```python
from build123d import *

# Parameters (mm, degrees)
F0_W     = 30
F0_H     = 72
F0_R     = 5
F1_DEPTH = 6
F2_R     = 1.25
F3_DEPTH = 1.5
F4_SIZE  = 0.5
F5_SIZE  = 1
F6_R     = 2
F7_W     = 34.31184
F7_H     = 14
F8_DEPTH = 4


with BuildPart() as f1:
    # F0 (on Front) → F1 (new body)
    with BuildSketch(Plane.XZ):
        with Locations((0, -28)):
            Rectangle(F0_W, F0_H)
        with Locations((0, -56)):
            Circle(F0_R, mode=Mode.SUBTRACT)
        with Locations((0, -28)):
            Circle(F0_R, mode=Mode.SUBTRACT)
        Circle(F0_R, mode=Mode.SUBTRACT)
    extrude(amount=-F1_DEPTH)

    # F2 (on Front) → F3 (join)
    with BuildSketch(Plane.XZ):
        with Locations((-13.51, 6.25)):
            Circle(F2_R)
        with Locations((0, -42)):
            Circle(F2_R)
    extrude(amount=F3_DEPTH)

    # F4
    f4_edges = [f1.edges().sort_by_distance(p)[0] for p in [
        (-14.76, -1.5, 6.25),
        (-1.25, -1.5, -42),
    ]]
    chamfer(f4_edges, length=F4_SIZE)

    # F5
    f5_edges = [f1.edges().sort_by_distance(p)[0] for p in [
        (-5, 6, -56),
        (-5, 6, -28),
        (-5, 6, 0),
        (-15, 6, -28),
        (0, 6, -64),
        (0, 6, 8),
        (15, 6, -28),
    ]]
    chamfer(f5_edges, length=F5_SIZE)

    # F6
    f6_edges = [f1.edges().sort_by_distance(p)[0] for p in [
        (-15, 2.5, 8),
        (15, 2.5, 8),
        (15, 2.5, -64),
        (-15, 2.5, -64),
    ]]
    fillet(f6_edges, radius=F6_R)

    # F7 (on Front) → F8 (cut)
    with BuildSketch(Plane.XZ):
        with Locations((5.65592, -14)):
            Rectangle(F7_W, F7_H)
    extrude(amount=-F8_DEPTH, mode=Mode.SUBTRACT)


solid = f1.part
```
Verification items for the finished model (mm, model axes). A direction names the side the tool comes from. Coordinates: 2 decimals unless noted, no trailing zeros. Order: outer loops, then holes, each group sorted by start corner. A loop starts at its lowest first (then second) coordinate and runs counter-clockwise, first axis right, second up. Notation, with made-up numbers: (-15.5, -30.75) -> (1.5, -30.75) arc R17 cw to (1.5, -21.75) -> close; hole circle Ø9 at (-24, -32). An arc over 180 degrees is marked (long way). Put each result on its own line as item: value. Start each with the question number.
1) Cross-section at A-A (z = 0). Enter the section's corners in (x, y).
2) Go/stop test with flat-tipped pins: pin 1 (13 mm diameter, centred on x = 0, z = -56, fed in from +Y); pin 2 (7 mm diameter, centred on x = 4.5, z = -17, fed in from -Y); pin 3 (16 mm diameter, centred on x = 0, z = 0, fed in from -Y). Record where each tip stops, or that it passes through.
3) Release check for a two-part mould opening along X. For faces 3 (the flat face through (0, 2, 8)), 4 (the flat face through (-11.5, 2, -14)), 5 (the cylindrical face through (-0.651, 2.465, -51.043)), 6 (the cylindrical face through (-14.43, 2.83, -63.4)) record: pulls with the +X half, pulls with the -X half, needs draft (parallel to the pull), parting line crosses it, or undercut.
4) Cross-section at C-C (y = 2.25). Enter the section's corners in (x, z).
5) Material ranges on L1, parallel to Z at x = 0, y = 3.25; L2, parallel to Z at x = -2.5, y = 3.5; L3, parallel to Z at x = 10, y = 2.25, recorded low to high.
6) Cross-section at D-D (z = -42). Enter the section's corners in (x, y), plus the area to 4 significant figures.
7) Cross-section at B-B (x = 0). State how many separate pieces and enclosed holes the cut face has, plus the area to 4 significant figures.
8) Tool access check on faces 1 (the flat face through (2, 2, -21)), 2 (the flat face through (0, -1.5, -42)). Record the directions out of +Z, -Z, +X, -X, +Y, -Y that give a thin tool (end or side, any length) a straight path to the whole face; none if there is none.
Geometry check:
1. outline: (-15, 0) -> (-5, 0) -> (-5, 5) -> (-6, 6) -> (-14, 6) -> (-15, 5) -> close; (5, 0) -> (15, 0) -> (15, 5) -> (14, 6) -> (6, 6) -> (5, 5) -> close
2. pin 1: stops at y = 6
2. pin 2: stops at y = 4
2. pin 3: stops at y = 0
3. face 3: needs draft
3. face 4: pulls with the +X half
3. face 5: undercut
3. face 6: pulls with the -X half
4. outline: (-15, -62) arc R2 ccw to (-13, -64) -> (13, -64) arc R2 ccw to (15, -62) -> (15, -21) -> (-11.5, -21) -> (-11.5, -7) -> (15, -7) -> (15, 6) arc R2 ccw to (13, 8) -> (-13, 8) arc R2 ccw to (-15, 6) -> close; hole circle Ø10 at (0, -56); hole circle Ø10 at (0, -28); hole circle Ø10 at (0, 0)
5. L1: z = -64 to -61, -51 to -33, -23 to -21, -7 to -5, 5 to 8
5. L2: z = -64 to -60.33, -51.67 to -32.33, -23.67 to -21, -7 to -4.33, 4.33 to 8
5. L3: z = -64 to -21, -7 to 8
6. outline: (-15, 0) -> (-1.25, 0) -> (-1.25, -1) -> (-0.75, -1.5) -> (0.75, -1.5) -> (1.25, -1) -> (1.25, 0) -> (15, 0) -> (15, 5) -> (14, 6) -> (-14, 6) -> (-15, 5) -> close
6. area: 182.5 mm^2
7. separate pieces: 4
7. enclosed holes: 0
7. area: 195.5 mm^2
8. face 1: +X, -Y
8. face 2: +Z, -Z, +X, -X, -Y
